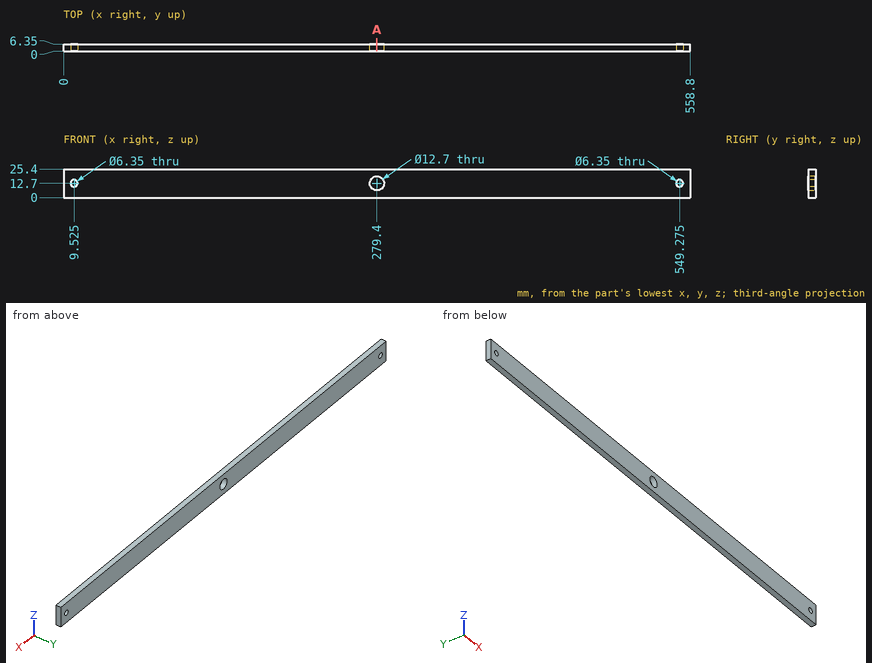
For this review, use the dimensioned drawing (mm, ordinates from the lowest corner) and the shaded views. Round coordinates to 2 decimals unless told otherwise and drop trailing zeros. Write each loop counter-clockwise with the first axis right and the second up, starting at its lowest first coordinate (ties: lowest second). Pieces come first, ordered by that corner, then holes. Notation, with made-up numbers: (58.5, 56) -> (88.5, 56) arc R34 ccw to (88.5, 94) -> close; hole circle Ø10 at (-21.75, 15). An arc over 180 degrees is marked (long way). Use one line per item in the form item = value.
Q1. Clearance check with a flat-ended pin moving along its axis: pin 1 Ø3 at (y, z) = (1, 20) entering from -X. State where the tip first meets the part, or that it passes through.
Resolved:
pin_1 = 0
Q2. Consider section A-A (x = 279.4). State the section outline as (y, z) points.
Resolved:
outline = (0, 0) -> (6.35, 0) -> (6.35, 6.35) -> (0, 6.35) -> close; (0, 19.05) -> (6.35, 19.05) -> (6.35, 25.4) -> (0, 25.4) -> close
Q3. To check wall thickness, follow probe 1 along X at (y, z) = (3.5, 12.7); probe 2 along X at (y, z) = (3.25, 11); probe 3 along Z at (x, y) = (279.4, 2.5). State the ranges of each line that lie inside material, in increasing order. Write a range as from..to.
Resolved:
probe_1 = 0..6.35, 12.7..273.05, 285.75..546.1, 552.45..558.8
probe_2 = 0..6.84, 12.21..273.28, 285.52..546.59, 551.96..558.8
probe_3 = 0..6.35, 19.05..25.4
